Geometry: final body of the model. Coordinates: model frame, mm. Face numbers are marked on the shaded views. A direction names the side the tool comes from. Coordinates: 2 decimals unless noted, no trailing zeros. Order: outer loops, then holes, each group sorted by start corner. A loop starts at its lowest first (then second) coordinate and runs counter-clockwise, first axis right, second up. Notation, with made-up numbers: (17, -20) -> (24, -20) arc R11 cw to (24, -16) -> close; hole circle Ø8 at (23.25, 14). An arc over 180 degrees is marked (long way). Use one line per item in the form item = value.
```python
from build123d import *

# Parameters (mm, degrees)
F1_DEPTH = 11
F3_DEPTH = 11


with BuildPart() as f1:
    # F0 (on Top) → F1 (new body)
    with BuildSketch(Plane.XY):
        with BuildLine():
            Line((-12.5, 3.5), (-7.0227744249, 3.5))
            ThreePointArc((-7.0227744249, 3.5), (-19, 0), (-7.0227744249, -3.5))
            Line((-7.0227744249, -3.5), (-12.5, -3.5))
            Line((-12.5, -3.5), (-12.5, 3.5))
        make_face()
        with BuildLine():
            ThreePointArc((7.0227744249, -3.5), (6, 0), (7.0227744249, 3.5))
            Line((7.0227744249, 3.5), (-7.0227744249, 3.5))
            ThreePointArc((-7.0227744249, 3.5), (-6.2609309093, 1.8231886576), (-6, 0))
            ThreePointArc((-6, 0), (-6.2609309093, -1.8231886576), (-7.0227744249, -3.5))
            Line((-7.0227744249, -3.5), (7.0227744249, -3.5))
        make_face()
        with BuildLine():
            Line((7.0227744249, 3.5), (12.5, 3.5))
            Line((12.5, 3.5), (12.5, -3.5))
            Line((12.5, -3.5), (7.0227744249, -3.5))
            ThreePointArc((7.0227744249, -3.5), (14.3231886576, -6.2390690907), (19, 0))
            ThreePointArc((19, 0), (14.3231886576, 6.2390690907), (7.0227744249, 3.5))
        make_face()
        with BuildLine():
            ThreePointArc((-6, 0), (-6.2609309093, 1.8231886576), (-7.0227744249, 3.5))
            Line((-7.0227744249, 3.5), (-12.5, 3.5))
            Line((-12.5, 3.5), (-12.5, -3.5))
            Line((-12.5, -3.5), (-7.0227744249, -3.5))
            ThreePointArc((-7.0227744249, -3.5), (-6.2609309093, -1.8231886576), (-6, 0))
        make_face()
        with BuildLine():
            Line((12.5, -3.5), (12.5, 3.5))
            Line((12.5, 3.5), (7.0227744249, 3.5))
            ThreePointArc((7.0227744249, 3.5), (6, 0), (7.0227744249, -3.5))
            Line((7.0227744249, -3.5), (12.5, -3.5))
        make_face()
    extrude(amount=F1_DEPTH)

    # F2 (on face) → F3 (cut, through all)
    with BuildSketch(Plane.XY.offset(11)):
        with BuildLine():
            ThreePointArc((-16.3729833462, -1), (-16.5, 0), (-16.3729833462, 1))
            Line((-16.3729833462, 1), (-18, 1))
            Line((-18, 1), (-18, -1))
            Line((-18, -1), (-16.3729833462, -1))
        make_face()
        with BuildLine():
            ThreePointArc((-16.3729833462, -1), (-11.9959828301, -3.9681187851), (-8.5, 0))
            ThreePointArc((-8.5, 0), (-11.9959828301, 3.9681187851), (-16.3729833462, 1))
            Line((-16.3729833462, 1), (-16, 1))
            Line((-16, 1), (-16, -1))
            Line((-16, -1), (-16.3729833462, -1))
        make_face()
        with BuildLine():
            Line((-16, 1), (-16.3729833462, 1))
            ThreePointArc((-16.3729833462, 1), (-16.5, 0), (-16.3729833462, -1))
            Line((-16.3729833462, -1), (-16, -1))
            Line((-16, -1), (-16, 1))
        make_face()
        with BuildLine():
            ThreePointArc((16.5, 0), (16.4681187851, 0.5040171699), (16.3729833462, 1))
            Line((16.3729833462, 1), (16, 1))
            Line((16, 1), (16, -1))
            Line((16, -1), (16.3729833462, -1))
            ThreePointArc((16.3729833462, -1), (16.4681187851, -0.5040171699), (16.5, 0))
        make_face()
        with BuildLine():
            Line((18, -1), (18, 1))
            Line((18, 1), (16.3729833462, 1))
            ThreePointArc((16.3729833462, 1), (16.4681187851, 0.5040171699), (16.5, 0))
            ThreePointArc((16.5, 0), (16.4681187851, -0.5040171699), (16.3729833462, -1))
            Line((16.3729833462, -1), (18, -1))
        make_face()
        with BuildLine():
            Line((16, 1), (16.3729833462, 1))
            ThreePointArc((16.3729833462, 1), (8.5, 0), (16.3729833462, -1))
            Line((16.3729833462, -1), (16, -1))
            Line((16, -1), (16, 1))
        make_face()
        with BuildLine():
            Line((-18, -1), (-18, 1))
            Line((-18, 1), (-18.9226162893, 1))
            ThreePointArc((-18.9226162893, 1), (-19, 0), (-18.9226162893, -1))
            Line((-18.9226162893, -1), (-18, -1))
        make_face()
        with BuildLine():
            Line((18.9226162893, 1), (18, 1))
            Line((18, 1), (18, -1))
            Line((18, -1), (18.9226162893, -1))
            ThreePointArc((18.9226162893, -1), (19, 0), (18.9226162893, 1))
        make_face()
        with BuildLine():
            ThreePointArc((18.9226162893, 1), (18.5872936506, 2.2792226771), (18, 3.4641016151))
            Line((18, 3.4641016151), (18, 1))
            Line((18, 1), (18.9226162893, 1))
        make_face()
        with BuildLine():
            Line((18, -1), (18, -3.4641016151))
            ThreePointArc((18, -3.4641016151), (18.5872936506, -2.2792226771), (18.9226162893, -1))
            Line((18.9226162893, -1), (18, -1))
        make_face()
        with BuildLine():
            Line((-18.9226162893, 1), (-18, 1))
            Line((-18, 1), (-18, 3.4641016151))
            ThreePointArc((-18, 3.4641016151), (-18.5872936506, 2.2792226771), (-18.9226162893, 1))
        make_face()
        with BuildLine():
            Line((-18, -3.4641016151), (-18, -1))
            Line((-18, -1), (-18.9226162893, -1))
            ThreePointArc((-18.9226162893, -1), (-18.5872936506, -2.2792226771), (-18, -3.4641016151))
        make_face()
    extrude(amount=-F3_DEPTH, mode=Mode.SUBTRACT)


solid = f1.part
```
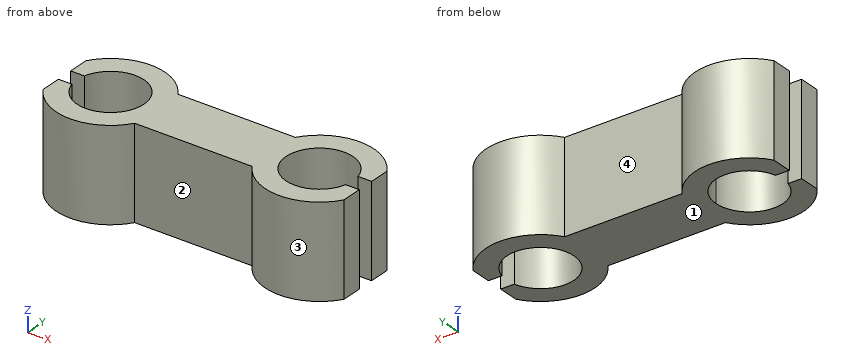
1) Access query for the marked faces 3 and 4. Directions: +Z, -Z, +X, -X, +Y, -Y. A direction counts if a zero-diameter tool reaches every point of the face in a straight line with its end or side. Return the directions, or none.
Results found:
face_3 = +Z, -Z, -Y
face_4 = +Z, -Z, +Y
2) Section D-D, the plane y = 5. Output: boundary loops of the cut face in (x, z).
Results found:
outline = (-16.65, 0) -> (-8.35, 0) -> (-8.35, 11) -> (-16.65, 11) -> close; (8.35, 0) -> (16.65, 0) -> (16.65, 11) -> (8.35, 11) -> close
3) Section A-A, the plane x = 12.5. Output: boundary loops of the cut face in (y, z), and give its area (3 significant figures).
Results found:
outline = (-6.5, 0) -> (-4, 0) -> (-4, 11) -> (-6.5, 11) -> close; (4, 0) -> (6.5, 0) -> (6.5, 11) -> (4, 11) -> close
area = 55.0 mm2
4) Material intervals for probe 1 along X at (y, z) = (2.5, 10.75); probe 2 along X at (y, z) = (2.25, 5.5); probe 3 along Y at (x, z) = (12.5, 6), sorted ascending. Write a range as from..to.
Results found:
probe_1 = -18..-15.62, -9.38..9.38, 15.62..18
probe_2 = -18..-15.81, -9.19..9.19, 15.81..18
probe_3 = -6.5..-4, 4..6.5
5) Pull-direction query (X, two-part tool) for the marked faces 1 and 2; classes: released by +X, released by -X, zero draft, split by the parting line, or undercut.
Results found:
face_1 = zero draft
face_2 = undercut
6) Section C-C, the plane z = 5.75. Output: boundary loops of the cut face in (x, y), and give its area (3 significant figures).
Results found:
outline = (-18, -3.46) arc R6.5 ccw to (-7.02, -3.5) -> (7.02, -3.5) arc R6.5 ccw to (18, -3.46) -> (18, -1) -> (16.37, -1) arc R4 cw (long way) to (16.37, 1) -> (18, 1) -> (18, 3.46) arc R6.5 ccw to (7.02, 3.5) -> (-7.02, 3.5) arc R6.5 ccw to (-18, 3.46) -> (-18, 1) -> (-16.37, 1) arc R4 cw (long way) to (-16.37, -1) -> (-18, -1) -> close
area = 238 mm2
7) Contact query for flat-ended pins moving along their axis: P1, Ø1.5, axis at x = 6, z = 2.5, coming from the -Y side; P2, Ø1.3, axis at x = 17, z = 8, coming from the +Y side; P3, Ø0.5, axis at x = 17, z = 6.5, coming from the -Y side. Output: stop coordinate, or through.
Results found:
P1 = -3.5
P2 = 5.24
P3 = -4.92
8) Section B-B, the plane y = -1.5. Output: boundary loops of the cut face in (x, z).
Results found:
outline = (-18, 0) -> (-16.21, 0) -> (-16.21, 11) -> (-18, 11) -> close; (-8.79, 0) -> (8.79, 0) -> (8.79, 11) -> (-8.79, 11) -> close; (16.21, 0) -> (18, 0) -> (18, 11) -> (16.21, 11) -> close
